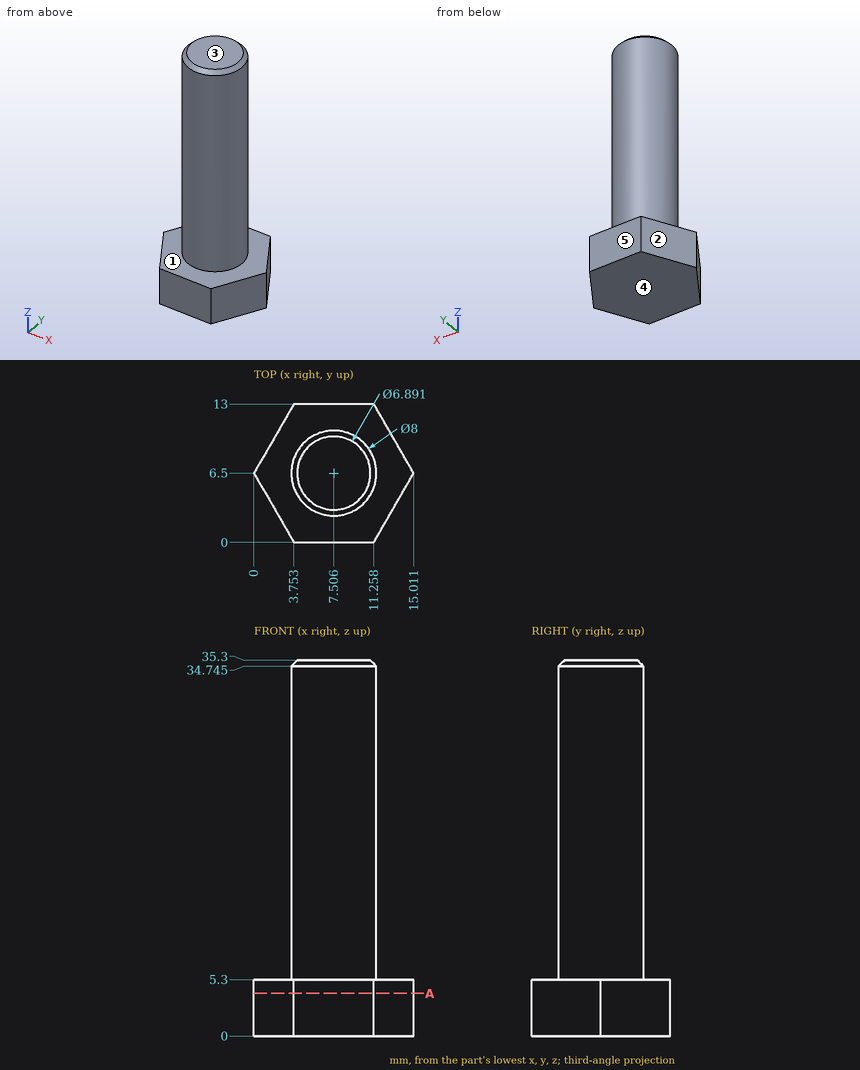
Source: three-view drawing plus pictorial views. Frame: mm from the lowest corner of the part. A direction names the side the tool comes from. Round coordinates to 2 decimals unless told otherwise and drop trailing zeros. Loops run counter-clockwise (first coordinate to the right, second up) from the corner with the lowest first, then second, coordinate; pieces in that order, holes last. Notation, with made-up numbers: M 75.25,49.25 L 99.25,49.25 A34 ccw 99.25,83.25 Z; hole C 83,59 d9. An arc over 180 degrees is marked long. Put each result on its own line as item: value. Start each with the question number.
(1) Set-up query: the marked faces 1 and 2. Return all of +Z, -Z, +X, -X, +Y, -Y with unobstructed straight access to the full face (end or side cutting, diameter ignored); none if empty.
(2) Contact query for flat-ended pins moving along their axis: pin 1 Ø5 at (x, z) = (12, 9.5) entering from +Y; pin 2 Ø5 at (y, z) = (5, 8) entering from +X; pin 3 Ø1.5 at (y, z) = (3.5, 16) entering from +X. Output: stop coordinate, or through.
(3) Material intervals for line 1 along Z through (x, y) = (12.5, 10.25); line 2 along Y through (x, z) = (7.5, 19); line 3 along X through (y, z) = (8.5, 31.5), sorted ascending. Write a range as [from, to].
(4) Section query A-A (z = 4). Return loops of the section in (x, y), then the cut area to 3 significant figures.
(5) Draft query along Z for the marked faces 3, 4 and 5. Return one class per face: +Z half, -Z half, draft (parallel to the pull), parting line (faces both ways), or undercut.
Findings below:
1. face 1: +Z
1. face 2: +Z, -Z, -X, +Y
2. pin 1: stops at y = 9.97
2. pin 2: stops at x = 11.51
2. pin 3: stops at x = 10.81
3. line 1: z = [0, 5.3]
3. line 2: y = [2.5, 10.5]
3. line 3: x = [4.04, 10.97]
4. outline: M 0,6.5 L 3.75,0 L 11.26,0 L 15.01,6.5 L 11.26,13 L 3.75,13 Z
4. area: 146 mm2
5. face 3: +Z half
5. face 4: -Z half
5. face 5: draft
